Read the model definition and answer for the solid it produces. Units are mm, in the model's axes. Face numbers are marked on the shaded views. A direction names the side the tool comes from. Round coordinates to 2 decimals unless told otherwise and drop trailing zeros. Loops run counter-clockwise (first coordinate to the right, second up) from the corner with the lowest first, then second, coordinate; pieces in that order, holes last. Notation, with made-up numbers: M 86.25,46 L 104.25,46 A23 cw 104.25,81 Z; hole C -24,-13.75 d5. An arc over 180 degrees is marked long. Answer as CSV lines item,"result".
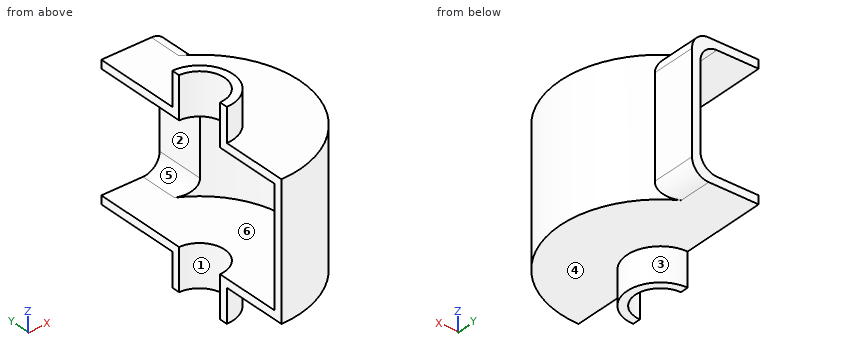
```python
from build123d import *

# Parameters (mm, degrees)
BOSS_EXTRUDE1_DEPTH = 25
BOSS_EXTRUDE3_DEPTH = 5
EXTRUDE_THIN2_START = -70
EXTRUDE_THIN2_DEPTH = 70
FILLET1_R           = 10


with BuildPart() as part:
    # Sketch1 → Boss-Extrude1 (new body)
    with BuildSketch(Plane.XY):
        with BuildLine():
            Line((0, -20), (0, -15))
            ThreePointArc((0, -15), (15, 0), (0, 15))
            Line((0, 15), (0, 20))
            ThreePointArc((0, 20), (20, 0), (0, -20))
        make_face()
    extrude(amount=BOSS_EXTRUDE1_DEPTH)


with BuildPart() as body_2:
    # Sketch3 → Boss-Extrude3 (new body)
    with BuildSketch(Plane.XY):
        with BuildLine():
            Line((0, -20), (0, -60))
            ThreePointArc((0, -60), (56.050341538, -21.409325386), (40, 44.72135955))
            Line((40, 44.72135955), (40, 72))
            Line((40, 72), (0, 72))
            Line((0, 72), (0, 60))
            Line((0, 60), (0, 20))
            ThreePointArc((0, 20), (20, 0), (0, -20))
        make_face()
    extrude(amount=BOSS_EXTRUDE3_DEPTH)


with BuildPart() as body_3:
    # Mirror5: mirrored copy
    add(part.part.mirror(Plane.XY.offset(-35)))


with BuildPart() as body_4:
    # Mirror5 2: mirrored copy
    add(body_2.part.mirror(Plane.XY.offset(-35)))


with BuildPart() as part_1:
    add(part.part)

    add(body_2.part)  # Extrude-Thin2 merges body 2

    add(body_4.part)  # Extrude-Thin2 merges body 4

    add(body_3.part)  # Extrude-Thin2 merges body 3
    # Sketch5 → Extrude-Thin2 (add)
    with BuildSketch(Plane.XY.offset(EXTRUDE_THIN2_START)):
        with BuildLine():
            ThreePointArc((0, -60), (56.050341538, -21.409325386), (40, 44.72135955))
            Line((40, 44.72135955), (40, 72))
            Line((40, 72), (35, 72))
            Line((35, 72), (35, 42.426406871))
            ThreePointArc((35, 42.426406871), (51.76124215, -18.594994247), (0, -55))
            Line((0, -55), (0, -60))
        make_face()
    extrude(amount=EXTRUDE_THIN2_DEPTH)

    # Fillet1
    fillet1_edges = [part_1.edges().sort_by_distance(p)[0] for p in [
        (40, 58.360679775, 5),
        (35, 57.213203436, -70),
        (35, 57.213203436, 0),
        (40, 58.360679775, -75),
    ]]
    fillet(fillet1_edges, radius=FILLET1_R)


solid = part_1.part
```
1) Straight lines are drawn through the part: line 1 (Z direction, x = 19, y = 50.5); line 2 (X direction, y = 1.5, z = -8); line 3 (Y direction, x = 46, z = -59). For each, find the intervals that lie inside material, in ascending order.
Evaluation:
line 1,"z = -75 to -70, 0 to 5"
line 2,"x = 54.98 to 59.98"
line 3,"y = -38.52 to -30.15, 30.15 to 38.52"
2) Find section D-D, the plane z = -80. Give the vertices of the cut face in (x, y), then the cut area to 3 significant figures.
Evaluation:
outline,"M 0,-20 A20 ccw 0,20 L 0,15 A15 cw 0,-15 Z"
area,"275 mm^2"
3) A tool of negligible diameter and unlimited length cuts with its end or side. For the marked faces 4, 5 and 6, from which of +Z, -Z, +X, -X, +Y, -Y can it reach the whole face along a straight path? Write none if from no direction.
Evaluation:
face 4,"-Z, +X"
face 5,"-X, +Y"
face 6,"-X"
4) Determine the mould class of the marked faces 1, 2 and 3 for opening direction Y: released by +Y, released by -Y, zero draft, split by the parting line, or undercut.
Evaluation:
face 1,"undercut"
face 2,"zero draft"
face 3,"split by the parting line"
5) Find section C-C, the plane x = 48.5. Give the vertices of the cut face in (y, z), then the cut area to 3 significant figures.
Evaluation:
outline,"M -35.32,-75 L 35.32,-75 L 35.32,5 L -35.32,5 Z; hole M -25.94,-70 L 25.94,-70 L 25.94,0 L -25.94,0 Z"
area,"2,020 mm^2"
6) Each of these flat-tipped pins is pushed along its axis until it touches: P1, Ø5, axis at y = 6.5, z = -32, coming from the +X side; P2, Ø4, axis at x = 51, y = 21, coming from the -Z side; P3, Ø10, axis at x = 53.5, y = 30, coming from the +Z side. Where does it stop, or does it pass through?
Evaluation:
P1,"stops at x = 59.87"
P2,"stops at z = -75"
P3,"stops at z = 5"
7) Find section A-A, the plane y = 0. Give the vertices of the cut face in (x, z), then the cut area to 3 significant figures.
Evaluation:
outline,"M 15,-95 L 20,-95 L 20,-75 L 60,-75 L 60,5 L 20,5 L 20,25 L 15,25 L 15,0 L 55,0 L 55,-70 L 15,-70 Z"
area,"1,000 mm^2"
8) Find section B-B, the plane x = 7.5. Give the vertices of the cut face in (y, z).
Evaluation:
outline,"M -59.53,-75 L -18.54,-75 L -18.54,-95 L -12.99,-95 L -12.99,-70 L -54.49,-70 L -54.49,0 L -12.99,0 L -12.99,25 L -18.54,25 L -18.54,5 L -59.53,5 Z; M 12.99,-95 L 18.54,-95 L 18.54,-75 L 72,-75 L 72,-70 L 12.99,-70 Z; M 12.99,0 L 72,0 L 72,5 L 18.54,5 L 18.54,25 L 12.99,25 Z"
